Design review of the part built by this model. Coordinates are the model's own, in mm. Round coordinates to 2 decimals unless told otherwise and drop trailing zeros. Write each loop counter-clockwise with the first axis right and the second up, starting at its lowest first coordinate (ties: lowest second). Pieces come first, ordered by that corner, then holes. Notation, with made-up numbers: M 38.25,17.5 L 68.25,17.5 A34 ccw 68.25,55.5 Z; hole C -30.5,87 d2. An arc over 180 degrees is marked long. One line per question, with ' | ' between items. Start each with the question number.
Item 1: Add section D-D, the plane x = -4. State the section outline as (y, z) points.
Item 2: Add section C-C, the plane y = 0. State the section outline as (x, z) points, and give its area (3 significant figures).
Item 3: Insertion check: pin 1 Ø1.4 at (x, y) = (6, 8) entering from +Z; pin 2 Ø2.5 at (x, y) = (0, -0.76) entering from -Z; pin 3 Ø4 at (y, z) = (-8, 8) entering from +X; pin 4 Ø1.5 at (x, y) = (-8.5, 2.5) entering from +Z. Each pin has a flat end and moves straight along its axis. Give the tip position at first contact, or say it passes through.
Item 4: Draft analysis for pull direction Y (two halves, no side actions). For faces 1 (the face through (-11.99, 0.53, 8.87)), 2 (the face through (4.95, -8.69, 8.92)), 3 (the face through (3, 11, 18)), state which applies: released by +Y, released by -Y, zero draft, split by the parting line, or undercut.
Item 5: Add section A-A, the plane x = 0. State the section outline as (y, z) points, and give its area (3 significant figures).
Item 6: Add section B-B, the plane z = 9. State the section outline as (x, y) points, and give its area (3 significant figures).
Item 7: For L1, parallel to Y at x = 0, z = 1.25; L2, parallel to X at y = -0.25, z = 7.5; L3, parallel to Y at x = -10.5, z = 5.25, list the stretches that pass through material, from the lowest coordinate up.
```python
from build123d import *

# Parameters (mm, degrees)
F0_R     = 10
F1_DEPTH = 3
F0_R_2   = 11
F2_DEPTH = 15
F0_R_3   = 12
F3_DEPTH = 18
F4_R     = 1.5
F5_DEPTH = 3
F7_DEPTH = 15


with BuildPart() as f1:
    # F0 (on Top) → F1 (new body)
    with BuildSketch(Plane.XY):
        Circle(F0_R)
    extrude(amount=F1_DEPTH)

    # F0 (on Top) → F2 (join)
    with BuildSketch(Plane.XY):
        Circle(F0_R_2)
        Circle(F0_R, mode=Mode.SUBTRACT)
    extrude(amount=F2_DEPTH)

    # F0 (on Top) → F3 (join)
    with BuildSketch(Plane.XY):
        Circle(F0_R_3)
        Circle(F0_R_2, mode=Mode.SUBTRACT)
    extrude(amount=F3_DEPTH)

    # F4 (on face) → F5 (cut)
    with BuildSketch(Plane.XY.offset(3)):
        with Locations((0, -0.7618688396)):
            Circle(F4_R)
    extrude(amount=-F5_DEPTH, mode=Mode.SUBTRACT)

    # F6 (on face) → F7 (cut)
    with BuildSketch(Plane.XY.offset(18)):
        with BuildLine():
            Line((0, 1.7320508076), (1.5, 2.5980762114))
            Line((1.5, 2.5980762114), (1.5, 10.8972473589))
            ThreePointArc((1.5, 10.8972473589), (0, 11), (-1.5, 10.8972473589))
            Line((-1.5, 10.8972473589), (-1.5, 2.5980762114))
            Line((-1.5, 2.5980762114), (0, 1.7320508076))
        make_face()
        with BuildLine():
            ThreePointArc((-1.5, 10.8972473589), (0, 11), (1.5, 10.8972473589))
            Line((1.5, 10.8972473589), (1.5, 11.5))
            Line((1.5, 11.5), (-1.5, 11.5))
            Line((-1.5, 11.5), (-1.5, 10.8972473589))
        make_face()
        with BuildLine():
            Line((-10.7092921435, 4.4509618943), (-10.1872930441, 4.1495855737))
            ThreePointArc((-10.1872930441, 4.1495855737), (-9.5262794416, 5.5), (-8.6872930441, 6.7476617851))
            Line((-8.6872930441, 6.7476617851), (-9.2092921435, 7.0490381057))
            Line((-9.2092921435, 7.0490381057), (-10.7092921435, 4.4509618943))
        make_face()
        with BuildLine():
            Line((-3, 0), (-1.5, 0.8660254038))
            Line((-1.5, 0.8660254038), (-1.5, 2.5980762114))
            Line((-1.5, 2.5980762114), (-8.6872930441, 6.7476617851))
            ThreePointArc((-8.6872930441, 6.7476617851), (-9.5262794416, 5.5), (-10.1872930441, 4.1495855737))
            Line((-10.1872930441, 4.1495855737), (-3, 0))
        make_face()
        with BuildLine():
            Line((-8.6872930441, -6.7476617851), (-1.5, -2.5980762114))
            Line((-1.5, -2.5980762114), (-1.5, -0.8660254038))
            Line((-1.5, -0.8660254038), (-3, 0))
            Line((-3, 0), (-10.1872930441, -4.1495855737))
            ThreePointArc((-10.1872930441, -4.1495855737), (-9.5262794416, -5.5), (-8.6872930441, -6.7476617851))
        make_face()
        with BuildLine():
            ThreePointArc((-1.5, -10.8972473589), (0, -11), (1.5, -10.8972473589))
            Line((1.5, -10.8972473589), (1.5, -2.5980762114))
            Line((1.5, -2.5980762114), (0, -1.7320508076))
            Line((0, -1.7320508076), (-1.5, -2.5980762114))
            Line((-1.5, -2.5980762114), (-1.5, -10.8972473589))
        make_face()
        with BuildLine():
            Line((1.5, -0.8660254038), (1.5, -2.5980762114))
            Line((1.5, -2.5980762114), (8.6872930441, -6.7476617851))
            ThreePointArc((8.6872930441, -6.7476617851), (9.5262794416, -5.5), (10.1872930441, -4.1495855737))
            Line((10.1872930441, -4.1495855737), (3, 0))
            Line((3, 0), (1.5, -0.8660254038))
        make_face()
        with BuildLine():
            Line((1.5, 2.5980762114), (1.5, 0.8660254038))
            Line((1.5, 0.8660254038), (3, 0))
            Line((3, 0), (10.1872930441, 4.1495855737))
            ThreePointArc((10.1872930441, 4.1495855737), (9.5262794416, 5.5), (8.6872930441, 6.7476617851))
            Line((8.6872930441, 6.7476617851), (1.5, 2.5980762114))
        make_face()
        with BuildLine():
            ThreePointArc((8.6872930441, 6.7476617851), (9.5262794416, 5.5), (10.1872930441, 4.1495855737))
            Line((10.1872930441, 4.1495855737), (10.7092921435, 4.4509618943))
            Line((10.7092921435, 4.4509618943), (9.2092921435, 7.0490381057))
            Line((9.2092921435, 7.0490381057), (8.6872930441, 6.7476617851))
        make_face()
        with BuildLine():
            ThreePointArc((10.1872930441, -4.1495855737), (9.5262794416, -5.5), (8.6872930441, -6.7476617851))
            Line((8.6872930441, -6.7476617851), (9.2092921435, -7.0490381057))
            Line((9.2092921435, -7.0490381057), (10.7092921435, -4.4509618943))
            Line((10.7092921435, -4.4509618943), (10.1872930441, -4.1495855737))
        make_face()
        with BuildLine():
            Line((-1.5, -11.5), (1.5, -11.5))
            Line((1.5, -11.5), (1.5, -10.8972473589))
            ThreePointArc((1.5, -10.8972473589), (0, -11), (-1.5, -10.8972473589))
            Line((-1.5, -10.8972473589), (-1.5, -11.5))
        make_face()
        with BuildLine():
            Line((-9.2092921435, -7.0490381057), (-8.6872930441, -6.7476617851))
            ThreePointArc((-8.6872930441, -6.7476617851), (-9.5262794416, -5.5), (-10.1872930441, -4.1495855737))
            Line((-10.1872930441, -4.1495855737), (-10.7092921435, -4.4509618943))
            Line((-10.7092921435, -4.4509618943), (-9.2092921435, -7.0490381057))
        make_face()
    extrude(amount=-F7_DEPTH, mode=Mode.SUBTRACT)


solid = f1.part
```
Computed values:
1) outline: M -11.31,0 L 11.31,0 L 11.31,18 L 10.25,18 L 10.25,15 L 9.17,15 L 9.17,3 L -9.17,3 L -9.17,15 L -10.25,15 L -10.25,18 L -11.31,18 Z
2) outline: M -12,0 L -1.29,0 L -1.29,3 L -10,3 L -10,15 L -11,15 L -11,18 L -12,18 Z; M 1.29,0 L 12,0 L 12,18 L 11,18 L 11,15 L 10,15 L 10,3 L 1.29,3 Z | area: 118 mm^2
3) pin 1: stops at z = 15 | pin 2: passes through | pin 3: stops at x = 10.39 | pin 4: stops at z = 3
4) face 1: split by the parting line | face 2: undercut | face 3: zero draft
5) outline: M -12,0 L -2.26,0 L -2.26,3 L -11.5,3 L -11.5,18 L -12,18 Z; M 0.74,0 L 12,0 L 12,18 L 11.5,18 L 11.5,3 L 0.74,3 Z | area: 78.0 mm^2
6) outline: C 0,0 d24; hole M -10.71,-4.45 L -9.21,-7.05 L -7.81,-6.24 A10 ccw -1.5,-9.89 L -1.5,-11.5 L 1.5,-11.5 L 1.5,-9.89 A10 ccw 7.81,-6.24 L 9.21,-7.05 L 10.71,-4.45 L 9.31,-3.64 A10 ccw 9.31,3.64 L 10.71,4.45 L 9.21,7.05 L 7.81,6.24 A10 ccw 1.5,9.89 L 1.5,11.5 L -1.5,11.5 L -1.5,9.89 A10 ccw -7.81,6.24 L -9.21,7.05 L -10.71,4.45 L -9.31,3.64 A10 ccw -9.31,-3.64 Z | area: 111 mm^2
7) L1: y = -12 to -2.26, 0.74 to 12 | L2: x = -12 to -10, 10 to 12 | L3: y = -5.81 to -4.81, -4.33 to 4.33, 4.81 to 5.81
